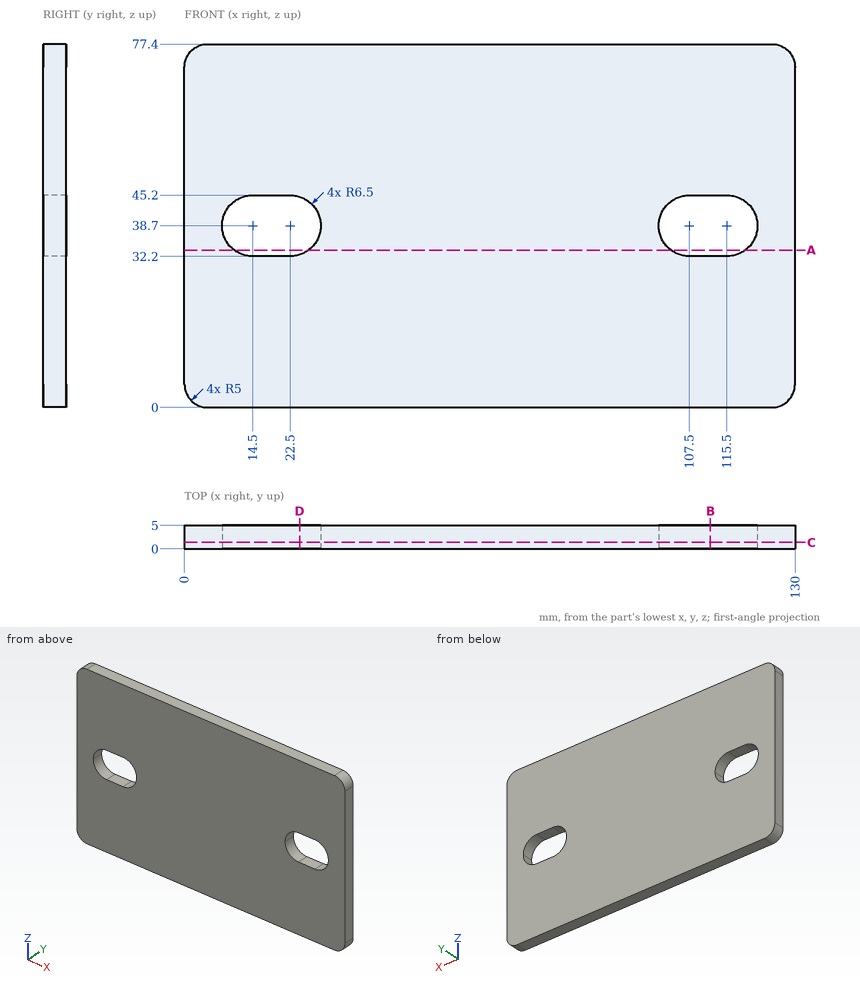
The drawing under review shows one solid part. Ordinate dimensions are in mm from its lowest x, y, z. Round coordinates to 2 decimals unless told otherwise and drop trailing zeros. Write each loop counter-clockwise with the first axis right and the second up, starting at its lowest first coordinate (ties: lowest second). Pieces come first, ordered by that corner, then holes. Notation, with made-up numbers: (68, -27.75) -> (73, -27.75) arc R28 cw to (73, 10.25) -> close; hole circle Ø10 at (63, 46). An arc over 180 degrees is marked (long way). Put each result on its own line as item: value.
Q1. Consider section B-B on x = 112. State the section outline as (y, z) points.
Determined:
outline: (0, 0) -> (5, 0) -> (5, 32.2) -> (0, 32.2) -> close; (0, 45.2) -> (5, 45.2) -> (5, 77.4) -> (0, 77.4) -> close
Q2. Consider section A-A on z = 33.5. State the section outline as (x, y) points.
Determined:
outline: (0, 0) -> (10.6, 0) -> (10.6, 5) -> (0, 5) -> close; (26.4, 0) -> (103.6, 0) -> (103.6, 5) -> (26.4, 5) -> close; (119.4, 0) -> (130, 0) -> (130, 5) -> (119.4, 5) -> close
Q3. Consider section C-C on y = 1.4. State the section outline as (x, z) points.
Determined:
outline: (0, 5) arc R5 ccw to (5, 0) -> (125, 0) arc R5 ccw to (130, 5) -> (130, 72.4) arc R5 ccw to (125, 77.4) -> (5, 77.4) arc R5 ccw to (0, 72.4) -> close; hole (14.5, 32.2) -> (22.5, 32.2) arc R6.5 ccw to (22.5, 45.2) -> (14.5, 45.2) arc R6.5 ccw to start; hole (107.5, 32.2) -> (115.5, 32.2) arc R6.5 ccw to (115.5, 45.2) -> (107.5, 45.2) arc R6.5 ccw to start
Q4. To check wall thickness, follow L1, parallel to X at y = 3.8, z = 44; L2, parallel to Z at x = 115, y = 1.9; L3, parallel to X at y = 2.9, z = 34. State the ranges of each line that lie inside material, in increasing order. Write a range as [from, to].
Determined:
L1: x = [0, 10.74], [26.26, 103.74], [119.26, 130]
L2: z = [0, 32.2], [45.2, 77.4]
L3: x = [0, 10.01], [26.99, 103.01], [119.99, 130]
Q5. Consider section D-D on x = 24.5. State the section outline as (y, z) points.
Determined:
outline: (0, 0) -> (5, 0) -> (5, 32.52) -> (0, 32.52) -> close; (0, 44.88) -> (5, 44.88) -> (5, 77.4) -> (0, 77.4) -> close
Q6. Clearance check with a flat-ended pin moving along its axis: pin 1 Ø1 at (y, z) = (1.5, 56) entering from -X. State where the tip first meets the part, or that it passes through.
Determined:
pin 1: stops at x = 0
